Could you check a few things on this model? Use its own coordinates, in mm. A direction names the side the tool comes from. Coordinates: 2 decimals unless noted, no trailing zeros. Loops run counter-clockwise (first coordinate to the right, second up) from the corner with the lowest first, then second, coordinate; pieces in that order, holes last. Notation, with made-up numbers: (5, 75) - (38, 75) arc R25 cw to (38, 108) - close; hole circle Ø2 at (12, 67.25). An arc over 180 degrees is marked (long way). One line per item, written item: value. Start each with the question number.
(1) If we section it at A-A on x = 0: Count the separate pieces of the cut face and the enclosed holes in it, then the cut area to 3 significant figures.
(2) If I drill on line 1 along Y through (x, z) = (-53.5, 24.5); line 2 along Z through (x, y) = (-58, 2.25); line 3 along X through (y, z) = (-7.5, 5.5), over which ranges is the centre line in solid material (lowest first)? Write a range as from..to.
(3) If we section it at C-C on y = -7: Write out the boundary of the cut face in (x, z).
(4) On a 3-axis mill with a long thin cutter (end or side, diameter ignored), from which of +Z, -Z, +X, -X, +Y, -Y can I reach the whole of each face in a straight line? I mean faces 5 (the face through (0, -4, 74.7)), 6 (the face through (0, -4, 42.5)), 7 (the face through (96.799, 4.098, 40.518)). Say none if no direction works.
(5) If we section it at B-B on z = 60.5: Write out the boundary of the cut face in (x, y).
(6) If we mould it in two halves opening along Y, with no side actions, what happens to faces 1 (the face through (0.54, -9.44, 7.76)), 2 (the face through (0, -4, 37.5)), 3 (the face through (0.54, -9.44, 39.97)), 4 (the face through (-6.605, -4.56, 72.165))? For each: pulls with the +Y half, pulls with the -Y half, needs draft (parallel to the pull), parting line crosses it, or undercut.
(7) I'm going to push flat-ended pins straight in: P1, Ø6, axis at x = 0, y = -7, coming from the +Z side; P2, Ø6, axis at x = 3.5, y = -7.5, coming from the -Z side; P3, Ø12, axis at x = 64, z = 45, coming from the -Y side. Where does each tip first touch, or does it pass through?
(8) If we section it at D-D on x = 79: Write out the boundary of the cut face in (y, z), then the cut area to 3 significant figures.
```python
from build123d import *

# Parameters (mm, degrees)
BOSS_EXTRUDE3_DEPTH = 80
BOSS_EXTRUDE2_START = -5.3
SKETCH2_R           = 2.5
BOSS_EXTRUDE2_DEPTH = 5
LPATTERN1_COUNT     = 3
LPATTERN1_PITCH     = 32.2
FILLET1_R           = 3
FILLET2_R           = 1


with BuildPart() as part:
    # Sketch3 → Boss-Extrude3 (new body)
    with BuildSketch(Plane.XY):
        Polygon((97.654693799, 0), (97.654693799, 5), (-76.347854423, 5), (-76.347854423, 0), (0, 0), align=None)
    extrude(amount=BOSS_EXTRUDE3_DEPTH)

    # Sketch2 → Boss-Extrude2 (add)
    with BuildSketch(Plane(origin=(0, 0, 0), x_dir=(-1, 0, 0), z_dir=(0, 0, -1)).offset(BOSS_EXTRUDE2_START)):
        with BuildLine():
            Line((-3.897114317, -9.25), (-9.237604307, 0))
            Line((-9.237604307, 0), (9.237604307, 0))
            Line((9.237604307, 0), (3.897114317, -9.25))
            ThreePointArc((3.897114317, -9.25), (0, -11.5), (-3.897114317, -9.25))
        make_face()
        with Locations((0, -7)):
            Circle(SKETCH2_R, mode=Mode.SUBTRACT)
    boss_extrude2 = extrude(amount=-BOSS_EXTRUDE2_DEPTH)

    # LPattern1: Boss-Extrude2 ×3
    with Locations(*[(0, 0, i * LPATTERN1_PITCH) for i in range(1, LPATTERN1_COUNT)]):
        add(boss_extrude2)

    # Fillet1
    fillet1_edges = [part.edges().sort_by_distance(p)[0] for p in [
        (10.653419688, 5, 80),
        (-76.347854423, 2.5, 80),
        (-76.347854423, 2.5, 0),
        (10.653419688, 5, 0),
        (97.654693799, 2.5, 0),
        (97.654693799, 2.5, 80),
        (-76.347854423, 5, 40),
        (97.654693799, 5, 40),
    ]]
    fillet(fillet1_edges, radius=FILLET1_R)

    # Fillet2
    fillet2_edges = [part.edges().sort_by_distance(p)[0] for p in [
        (97.654693799, 0, 40),
        (10.653419688, 0, 0),
        (-76.347854423, 0, 40),
        (10.653419688, 0, 80),
        (96.776014142, 0, 0.878679656),
        (-75.469174766, 0, 0.878679656),
        (-75.469174766, 0, 79.121320344),
        (96.776014142, 0, 79.121320344),
    ]]
    fillet(fillet2_edges, radius=FILLET2_R)


solid = part.part
```
Values:
1. separate pieces: 4
1. enclosed holes: 0
1. area: 493 mm2
2. line 1: y = 0..5
2. line 2: z = 0.01..79.99
2. line 3: x = -4.91..-2.45, 2.45..4.91
3. outline: (-5.2, 5.3) - (-2.5, 5.3) - (-2.5, 10.3) - (-5.2, 10.3) - close; (-5.2, 37.5) - (-2.5, 37.5) - (-2.5, 42.5) - (-5.2, 42.5) - close; (-5.2, 69.7) - (-2.5, 69.7) - (-2.5, 74.7) - (-5.2, 74.7) - close; (2.5, 5.3) - (5.2, 5.3) - (5.2, 10.3) - (2.5, 10.3) - close; (2.5, 37.5) - (5.2, 37.5) - (5.2, 42.5) - (2.5, 42.5) - close; (2.5, 69.7) - (5.2, 69.7) - (5.2, 74.7) - (2.5, 74.7) - close
4. face 5: +Z, +X, -X, -Y
4. face 6: +X, -X, -Y
4. face 7: +Z, -Z, +X, +Y
5. outline: (-76.35, 1) arc R1 ccw to (-75.35, 0) - (96.65, 0) arc R1 ccw to (97.65, 1) - (97.65, 2) arc R3 ccw to (94.65, 5) - (-73.35, 5) arc R3 ccw to (-76.35, 2) - close
6. face 1: undercut
6. face 2: needs draft
6. face 3: undercut
6. face 4: pulls with the -Y half
7. P1: stops at z = 74.7
7. P2: stops at z = 5.3
7. P3: stops at y = 0
8. outline: (0, 1) arc R1 ccw to (1, 0) - (2, 0) arc R3 ccw to (5, 3) - (5, 77) arc R3 ccw to (2, 80) - (1, 80) arc R1 ccw to (0, 79) - close
8. area: 396 mm2
